```python
from build123d import *

# Parameters (mm, degrees)
BASEBOSS_EXTRUDE1_DEPTH = 2
SKETCH3_W               = 8.636942675
SKETCH3_H               = 1
BOSS_EXTRUDE1_DEPTH     = 0.5
SKETCH4_W               = 8.636942675
SKETCH4_H               = 1
BOSS_EXTRUDE2_DEPTH     = 0.5
CHAMFER1_SIZE           = 0.5
CHAMFER2_SIZE           = 0.5


# Some blends are built 0.0001 mm under size
with BuildPart() as part:
    # Sketch1 → BaseBoss-Extrude1 (new body)
    with BuildSketch(Plane.XY):
        with BuildLine():
            Line((19.925716198, 10.915607247), (28.562658873, 10.915607247))
            ThreePointArc((28.562658873, 10.915607247), (35.562658873, 3.915607247), (28.562658873, -3.084392753))
            Line((28.562658873, -3.084392753), (19.925716198, -3.084392753))
            ThreePointArc((19.925716198, -3.084392753), (12.925716198, 3.915607247), (19.925716198, 10.915607247))
        make_face()
        with BuildLine():
            Line((20.244187536, 8.915607247), (28.244187536, 8.915607247))
            ThreePointArc((28.244187536, 8.915607247), (33.244187536, 3.915607247), (28.244187536, -1.084392753))
            Line((28.244187536, -1.084392753), (20.244187536, -1.084392753))
            ThreePointArc((20.244187536, -1.084392753), (15.244187536, 3.915607247), (20.244187536, 8.915607247))
        make_face(mode=Mode.SUBTRACT)
    extrude(amount=BASEBOSS_EXTRUDE1_DEPTH)

    # Sketch3 → Boss-Extrude1 (add)
    with BuildSketch(Plane.XZ.offset(-8.915607247)):
        with Locations((24.244187536, 0.9)):
            Rectangle(SKETCH3_W, SKETCH3_H)
    extrude(amount=BOSS_EXTRUDE1_DEPTH)

    # Sketch4 → Boss-Extrude2 (add)
    with BuildSketch(Plane(origin=(0, -1.084392753, 0), x_dir=(1, 0, 0), z_dir=(0, 1, 0))):
        with Locations((24.244187536, -1)):
            Rectangle(SKETCH4_W, SKETCH4_H)
    extrude(amount=BOSS_EXTRUDE2_DEPTH)

    # Chamfer1
    # the kernel refuses this chamfer: 0.5 mm, written as the material it takes off along each edge
    with BuildSketch(Plane(origin=(28.562658873, -0.584392753, -0.785841494), x_dir=(0.02749587661058907, -0.9996219169112965, 0), z_dir=(0, 0, 1))) as chamfer1_piece_1_section:
        Polygon((CHAMFER1_SIZE * 0.999621916911, -CHAMFER1_SIZE * 0.0274958766106), (-CHAMFER1_SIZE * 0.0274958766106, -CHAMFER1_SIZE * 0.999621916911), (0, 0), align=None)
    chamfer1_piece_1 = extrude(amount=3.571682988, mode=Mode.PRIVATE)
    chamfer1_piece_1 = chamfer1_piece_1 & Plane(origin=(28.244187536, 3.915607247, 1), x_dir=(0, 1, 0), z_dir=(0, 0, -1)) * Cylinder(5, 10, mode=Mode.PRIVATE)
    add(chamfer1_piece_1, mode=Mode.SUBTRACT)
    with BuildSketch(Plane(origin=(19.925716198, -0.584392753, 2.785841494), x_dir=(-0.02749587661058907, -0.9996219169112965, 0), z_dir=(0, 0, -1))) as chamfer1_piece_2_section:
        Polygon((CHAMFER1_SIZE * 0.999621916911, -CHAMFER1_SIZE * 0.0274958766106), (-CHAMFER1_SIZE * 0.0274958766106, -CHAMFER1_SIZE * 0.999621916911), (0, 0), align=None)
    chamfer1_piece_2 = extrude(amount=3.571682988, mode=Mode.PRIVATE)
    chamfer1_piece_2 = chamfer1_piece_2 & Plane(origin=(20.244187536, 3.915607247, 1), x_dir=(0, -1, 0), z_dir=(0, 0, -1)) * Cylinder(5, 10, mode=Mode.PRIVATE)
    add(chamfer1_piece_2, mode=Mode.SUBTRACT)
    with BuildSketch(Plane(origin=(28.562658873, 8.415607247, 2.685841494), x_dir=(0.0274958766105891, 0.9996219169112968, 0), z_dir=(0, 0, -1))) as chamfer1_piece_3_section:
        Polygon((CHAMFER1_SIZE * 0.999621916911, -CHAMFER1_SIZE * 0.0274958766106), (-CHAMFER1_SIZE * 0.0274958766106, -CHAMFER1_SIZE * 0.999621916911), (0, 0), align=None)
    chamfer1_piece_3 = extrude(amount=3.571682988, mode=Mode.PRIVATE)
    chamfer1_piece_3 = chamfer1_piece_3 & Plane(origin=(28.244187536, 3.915607247, 0.9), x_dir=(0, 1, 0), z_dir=(0, 0, -1)) * Cylinder(5, 10, mode=Mode.PRIVATE)
    add(chamfer1_piece_3, mode=Mode.SUBTRACT)
    with BuildSketch(Plane(origin=(19.925716198, 8.415607247, -0.885841494), x_dir=(-0.0274958766105891, 0.9996219169112968, 0), z_dir=(0, 0, 1))) as chamfer1_piece_4_section:
        Polygon((CHAMFER1_SIZE * 0.999621916911, -CHAMFER1_SIZE * 0.0274958766106), (-CHAMFER1_SIZE * 0.0274958766106, -CHAMFER1_SIZE * 0.999621916911), (0, 0), align=None)
    chamfer1_piece_4 = extrude(amount=3.571682988, mode=Mode.PRIVATE)
    chamfer1_piece_4 = chamfer1_piece_4 & Plane(origin=(20.244187536, 3.915607247, 0.9), x_dir=(0, -1, 0), z_dir=(0, 0, -1)) * Cylinder(5, 10, mode=Mode.PRIVATE)
    add(chamfer1_piece_4, mode=Mode.SUBTRACT)

    # Chamfer2
    chamfer2_edges = [part.edges().sort_by_distance(p)[0] for p in [
        (24.244187536, -0.584392753, 0.5),
        (24.244187536, 8.415607247, 0.4),
        (24.244187536, 8.415607247, 1.4),
        (24.244187536, -0.584392753, 1.5),
    ]]
    chamfer(chamfer2_edges, length=CHAMFER2_SIZE - 0.0001)  # a hair under: the kernel refuses the full size


solid = part.part
```
Part model, mm, in its own coordinate system. Give positions to 0.01 mm unless a question says otherwise; leave off trailing zeros. Write each loop counter-clockwise with the first axis right and the second up, starting at its lowest first coordinate (ties: lowest second). Pieces come first, ordered by that corner, then holes. Notation, with made-up numbers: (87, 4) -> (117, 4) arc R19 ccw to (117, 41) -> close; hole circle Ø10 at (86, 7.5). An arc over 180 degrees is marked (long way). Put each result on its own line as item: value. Start each with the question number.
Item 1: Pull direction Y, two halves, no side cores. Call faces 1 (the face through (33.243, 4.026, 0.986)), 2 (the face through (25.14, -1.24, 0)), 3 (the face through (15.245, 3.806, 0.986)), 4 (the face through (12.927, 3.762, 0.986)): pulls with the +Y half, pulls with the -Y half, needs draft (parallel to the pull), parting line crosses it, or undercut.
Item 2: Wall check: L1, parallel to Y at x = 22.25, z = 1.65; L2, parallel to X at y = 7.25, z = 0.15; L3, parallel to X at y = 5.25, z = 1.65. Give the ranges that are in metal, low to high. Write a range as [from, to].
Item 3: Cut at A-A (z = 1.75). List the corners of the cut face in (x, y).
Item 4: Cut at D-D (x = 18.75). List the corners of the cut face in (y, z).
Item 5: Cut at C-C (y = 6.75). List the corners of the cut face in (x, z).
Answer list:
1. face 1: undercut
1. face 2: needs draft
1. face 3: undercut
1. face 4: parting line crosses it
2. L1: y = [-3.08, -1.08], [8.92, 10.92]
2. L2: x = [13.77, 16.52], [31.97, 34.72]
2. L3: x = [13.05, 15.43], [33.06, 35.43]
3. outline: (19.93, -3.08) -> (28.56, -3.08) arc R7 ccw to (28.56, 10.92) -> (19.93, 10.92) arc R7 ccw to start; hole (20.24, -1.08) -> (28.24, -1.08) arc R5 ccw to (28.24, 8.92) -> (20.24, 8.92) arc R5 ccw to start
4. outline: (-2.98, 0) -> (-0.86, 0) -> (-0.86, 2) -> (-2.98, 2) -> close; (8.69, 0) -> (10.82, 0) -> (10.82, 2) -> (8.69, 2) -> close
5. outline: (13.53, 0) -> (16.13, 0) -> (16.13, 2) -> (13.53, 2) -> close; (32.36, 0) -> (34.96, 0) -> (34.96, 2) -> (32.36, 2) -> close
